Can you work these out from the model? Positions are in its coordinate system, mm. A direction names the side the tool comes from. Give positions to 0.01 mm unless a question says otherwise; leave off trailing zeros. Order: outer loops, then holes, each group sorted by start corner. A loop starts at its lowest first (then second) coordinate and runs counter-clockwise, first axis right, second up. Notation, with made-up numbers: M 13,25 L 33,25 A32 cw 33,62 Z; hole C 75.5,85.25 d6. An arc over 180 degrees is marked long. Use one line per item in the form item = value. Start each with the question number.
1. For faces 1 (the face through (1.512, -1.493, 2.602)), 2 (the face through (1.512, 0.493, 2.602)), 3 (the face through (-9.4, -0.5, 0)), which set-ups out of +Z, -Z, +X, -X, +Y, -Y let a thin tool reach every point of the face, with its end or its side?
2. I want a section at A-A, the plane x = -4. List the corners of the cut face in (y, z) for me, and give its area (3 significant figures).
3. I need wall thicknesses on L1, parallel to Y at x = 14.5, z = 4; L2, parallel to X at y = -0.6, z = 6; L3, parallel to X at y = -0.4, z = 1. Which ranges of each line are inside material? Lowest first, please.
4. I want a section at B-B, the plane y = -1.4. List the corners of the cut face in (x, z) for me.
5. Will these pins go through, and if not, where does the flat tip stop? P1, Ø4, axis at x = -5, z = 3.5, coming from the +Y side; P2, Ø3.5, axis at x = 11.5, z = 4, coming from the -Y side.
```python
from build123d import *

# Parameters (mm, degrees)
F0_R     = 1.016
F1_DEPTH = 1
F2_DEPTH = 2
F3_DEPTH = 1


with BuildPart() as f1:
    # F0 (on Front) → F1 (new body)
    with BuildSketch(Plane.XZ):
        with BuildLine():
            Line((22.5296217646, 7), (5.0296217646, 7))
            Line((5.0296217646, 7), (5.0296217646, 0))
            Line((5.0296217646, 0), (25.0296217646, 0))
            Line((25.0296217646, 0), (25.0296217646, 4.5))
            ThreePointArc((25.0296217646, 4.5), (24.2973887176, 6.267766953), (22.5296217646, 7))
        make_face()
        with BuildLine():
            Line((-0.5277903524, 7), (-20.5277903524, 7))
            Line((-20.5277903524, 7), (-20.5277903524, 2.5))
            ThreePointArc((-20.5277903524, 2.5), (-19.7955573054, 0.732233047), (-18.0277903524, 0))
            Line((-18.0277903524, 0), (-0.5277903524, 0))
            Line((-0.5277903524, 0), (-0.5277903524, 7))
        make_face()
        with BuildLine():
            add(Edge.make_bspline(
                [(-0.5277903524, 7), (0.2936347767, 5.4160328527), (2.4654319937, 3.2330255819), (4.0015688672, 5.4588735962), (5.0296217646, 7)],
                knots=[0, 0, 0, 0, 0.503153471, 1, 1, 1, 1], degree=3))
            Line((-0.5277903524, 7), (-0.5277903524, 0))
            add(Edge.make_bspline(
                [(-0.5277903524, 0), (0.3996940581, 1.0133841191), (2.2540528119, 3.0394852076), (4.104635181, 1.0129391145), (5.0296217646, 0)],
                knots=[0, 0, 0, 0, 0.5001646338, 1, 1, 1, 1], degree=3))
            Line((5.0296217646, 0), (5.0296217646, 7))
        make_face()
        with Locations((2.3182034492, 3.2204561867)):
            Circle(F0_R, mode=Mode.SUBTRACT)
    extrude(amount=F1_DEPTH)

    # F0 (on Front) → F2 (join)
    with BuildSketch(Plane.XZ):
        with Locations((2.3182034492, 3.2204561867)):
            Circle(F0_R)
    extrude(amount=F2_DEPTH)

    # F0 (on Front) → F3 (join)
    with BuildSketch(Plane.XZ):
        with Locations((2.3182034492, 3.2204561867)):
            Circle(F0_R)
    extrude(amount=-F3_DEPTH)


solid = f1.part
```
Check result:
q1.face_1 = -Y
q1.face_2 = +Y
q1.face_3 = -Z, +X, -X, +Y, -Y
q2.outline = M -1,0 L 0,0 L 0,7 L -1,7 Z
q2.area = 7.00 mm2
q3.L1 = -1 to 0
q3.L2 = -20.53 to 0.07, 4.35 to 24.53
q3.L3 = -20.03 to 0.42, 4.08 to 25.03
q4.outline = C 2.32,3.22 d2.03
q5.P1 = 0
q5.P2 = -1
